Input: dimensioned drawing with shaded views. Units: mm. Origin: part minimum x, y, z. Round coordinates to 2 decimals unless told otherwise and drop trailing zeros. Loops run counter-clockwise (first coordinate to the right, second up) from the corner with the lowest first, then second, coordinate; pieces in that order, holes last. Notation, with made-up numbers: M 1,25.25 L 17,25.25 A18 ccw 17,59.25 Z; hole C -35.75,-17.75 d10. An arc over 180 degrees is marked long. Put each result on its own line as item: value. Start each with the question number.
1) Section B-B on x = 59. Output: boundary loops of the cut face in (y, z), plus the area to 3 significant figures.
2) Section C-C on y = 42. Output: boundary loops of the cut face in (x, z).
3) Pin query (flat end, axial travel): pin 1 (1.6 mm diameter, centred on y = 8, z = 2, fed in from +X); pin 2 (6 mm diameter, centred on x = 101, y = 39.5, fed in from +Z); pin 3 (0.6 mm diameter, centred on x = 108, y = 32.5, fed in from -Z); pin 4 (1 mm diameter, centred on x = 104.5, z = 2, fed in from -Y). Return the tip coordinate at first contact, or that it passes through.
4) Line query: probe 1 along X at (y, z) = (9, 2.6); probe 2 along Z at (x, y) = (90, 5); probe 3 along X at (y, z) = (34, 0.9). Output: solid intervals per line, ascending.
5) Section A-A on z = 2.2. Output: boundary loops of the cut face in (x, y).
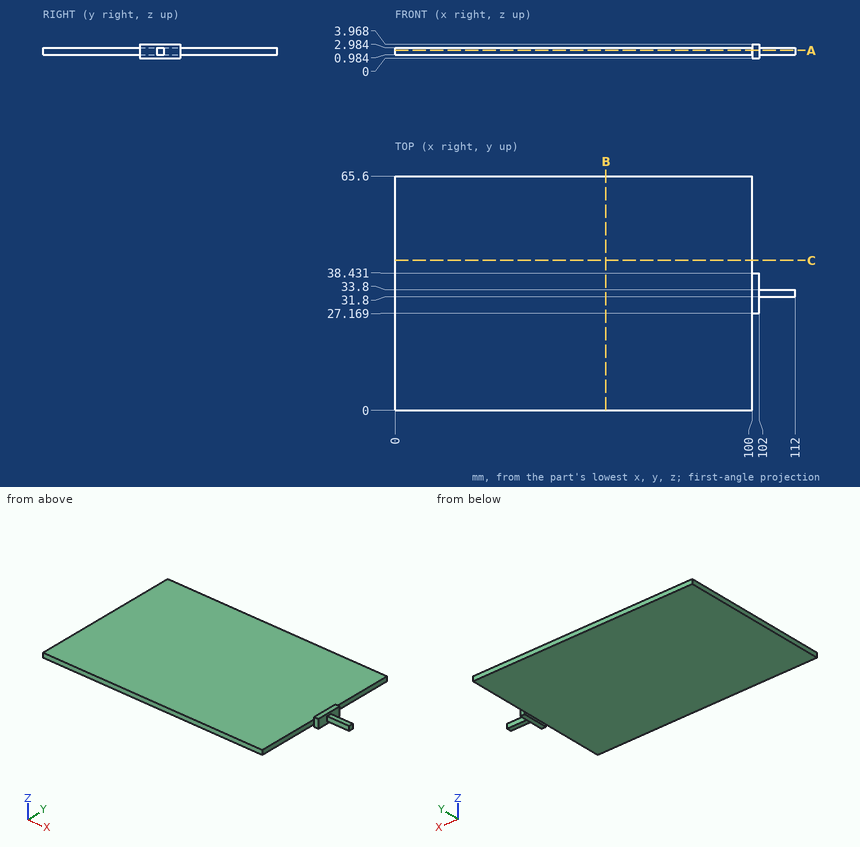
Geometry results:
1. outline: M 0,0.98 L 65.6,0.98 L 65.6,2.98 L 0,2.98 Z
1. area: 131 mm²
2. outline: M 0,0.98 L 100,0.98 L 100,2.98 L 0,2.98 Z
3. pin 1: stops at x = 100
3. pin 2: stops at z = 3.97
3. pin 3: stops at z = 0.98
3. pin 4: stops at y = 31.8
4. probe 1: x = 0 to 100
4. probe 2: z = 0.98 to 2.98
4. probe 3: x = 100 to 102
5. outline: M 0,0 L 100,0 L 100,27.17 L 102,27.17 L 102,31.8 L 112,31.8 L 112,33.8 L 102,33.8 L 102,38.43 L 100,38.43 L 100,65.6 L 0,65.6 Z
